Source: CAD feature listing. Evaluate the final solid. Frame: model axes, mm. Round coordinates to 2 decimals unless told otherwise and drop trailing zeros. Order: outer loops, then holes, each group sorted by start corner. A loop starts at its lowest first (then second) coordinate and runs counter-clockwise, first axis right, second up.
```python
from build123d import *

# Parameters (mm, degrees)
SKETCH2_R           = 1.15
SKETCH2_R_2         = 0.85
BOSS_EXTRUDE1_DEPTH = 1.8


with BuildPart() as part:
    # Sketch2 → Boss-Extrude1 (new body)
    with BuildSketch(Plane.XY):
        Circle(SKETCH2_R)
        Circle(SKETCH2_R_2, mode=Mode.SUBTRACT)
        with BuildLine():
            Line((-1.15, 2), (-1.15, 0))
            ThreePointArc((-1.15, 0), (0, 1.15), (1.15, 0))
            ThreePointArc((1.15, 0), (0.813172798, -0.813172798), (0, -1.15))
            Line((0, -1.15), (4.889316376, -1.15))
            Line((4.889316376, -1.15), (12.47489452, 2))
            Line((12.47489452, 2), (-1.15, 2))
        make_face()
    extrude(amount=BOSS_EXTRUDE1_DEPTH)


solid = part.part
```
1. Section B-B on z = 1.65. Return loops of the section in (x, y), plus the area to 3 significant figures.
2. Line query: line 1 along Y through (x, z) = (0, 1.35); line 2 along X through (y, z) = (0.75, 1.4); line 3 along X through (y, z) = (-0.2, 1.7). Output: solid intervals per line, ascending.
3. Section A-A on y = 0.3. Return loops of the section in (x, z), plus the area to 3 significant figures.
4. Section D-D on x = 8.5. Return loops of the section in (y, z).
5. Section C-C on y = -0.5. Return loops of the section in (x, z), plus the area to 3 significant figures.
Result:
1. outline: (-1.15, 0) arc R1.15 ccw to (0, -1.15) - (4.89, -1.15) - (12.47, 2) - (-1.15, 2) - close; hole circle Ø1.7 at (0, 0)
1. area: 28.4 mm2
2. line 1: y = -1.15 to -0.85, 0.85 to 2
2. line 2: x = -1.15 to -0.4, 0.4 to 9.46
2. line 3: x = -1.13 to -0.83, 0.83 to 7.18
3. outline: (-1.15, 0) - (-0.8, 0) - (-0.8, 1.8) - (-1.15, 1.8) - close; (0.8, 0) - (8.38, 0) - (8.38, 1.8) - (0.8, 1.8) - close
3. area: 14.3 mm2
4. outline: (0.35, 0) - (2, 0) - (2, 1.8) - (0.35, 1.8) - close
5. outline: (-1.04, 0) - (-0.69, 0) - (-0.69, 1.8) - (-1.04, 1.8) - close; (0.69, 0) - (6.45, 0) - (6.45, 1.8) - (0.69, 1.8) - close
5. area: 11.0 mm2
